Verification items for the finished model (mm, model axes). A direction names the side the tool comes from. Coordinates: 2 decimals unless noted, no trailing zeros. One line per item, written item: value.
```python
from build123d import *

# Parameters (mm, degrees)
F1_DEPTH = 10.16
F2_DEPTH = 12.7


with BuildPart() as f1:
    # F0 (on Front) → F1 (new body)
    with BuildSketch(Plane.XZ):
        with BuildLine():
            ThreePointArc((4.0007179822, 15.285099137), (12.5070249084, 9.654756752), (15.8, 0))
            ThreePointArc((15.8, 0), (-9.7296675451, -12.4488380768), (-3.8169075269, 15.332032381))
            Line((-3.8169075269, 15.332032381), (-3.8169075269, 20.4823272433))
            ThreePointArc((-3.8169075269, 20.4823272433), (-13.314831815, -16.0252852116), (20.834934902, 0))
            ThreePointArc((20.834934902, 0), (16.0849185744, 13.2427303388), (4.0007179822, 20.4472190774))
            Line((4.0007179822, 20.4472190774), (4.0007179822, 15.285099137))
        make_face()
        with BuildLine():
            ThreePointArc((-3.8169075269, 15.332032381), (0.0948538519, 15.7997152742), (4.0007179822, 15.285099137))
            Line((4.0007179822, 15.285099137), (4.0007179822, 20.4472190774))
            ThreePointArc((4.0007179822, 20.4472190774), (2.2310298491, 20.7151398302), (0.4448769206, 20.8301847543))
            Line((0.4448769206, 20.8301847543), (0.1276157176, 20.4966947721))
            Line((0.1276157176, 20.4966947721), (1.8328047784, 18.239185214))
            Line((1.8328047784, 18.239185214), (1.1116877884, 18.239185214))
            Line((1.1116877884, 18.239185214), (-0.2777255205, 20.0982431868))
            Line((-0.2777255205, 20.0982431868), (-0.7255529506, 19.7101260807))
            Line((-0.7255529506, 19.7101260807), (-0.7255529506, 18.239185214))
            Line((-0.7255529506, 18.239185214), (-1.3146182626, 18.239185214))
            Line((-1.3146182626, 18.239185214), (-1.3146182626, 20.7934194205))
            ThreePointArc((-1.3146182626, 20.7934194205), (-2.5704734618, 20.6757630707), (-3.8169075269, 20.4823272433))
            Line((-3.8169075269, 20.4823272433), (-3.8169075269, 15.332032381))
        make_face()
        with BuildLine():
            ThreePointArc((0.4448769206, 20.8301847543), (2.2310298491, 20.7151398302), (4.0007179822, 20.4472190774))
            Line((4.0007179822, 20.4472190774), (4.0007179822, 26.7865807325))
            Line((4.0007179822, 26.7865807325), (-3.8169075269, 26.7865807325))
            Line((-3.8169075269, 26.7865807325), (-3.8169075269, 20.4823272433))
            ThreePointArc((-3.8169075269, 20.4823272433), (-2.5704734618, 20.6757630707), (-1.3146182626, 20.7934194205))
            Line((-1.3146182626, 20.7934194205), (-1.3146182626, 23.8232487851))
            Line((-1.3146182626, 23.8232487851), (-0.7255529506, 23.8232487851))
            Line((-0.7255529506, 23.8232487851), (-0.7255529506, 20.861846369))
            add(Edge.make_bspline(
                [(-0.7255529506, 20.861846369), (-0.7255529506, 20.843060722), (-0.7258157075, 20.8222886334)],
                knots=[0, 0, 0, 0.0956718037, 0.0956718037, 0.0956718037], degree=2))
            ThreePointArc((-0.7258157075, 20.8222886334), (-0.4874986739, 20.8292308407), (-0.2491178041, 20.833445531))
            Line((-0.2491178041, 20.833445531), (1.0140843741, 22.172028671))
            Line((1.0140843741, 22.172028671), (1.7214220586, 22.172028671))
            Line((1.7214220586, 22.172028671), (0.4448769206, 20.8301847543))
        make_face()
    extrude(amount=F1_DEPTH)

    # F0 (on Front) → F2 (join)
    with BuildSketch(Plane.XZ):
        with BuildLine():
            ThreePointArc((4.0007179822, 15.285099137), (12.5070249084, 9.654756752), (15.8, 0))
            ThreePointArc((15.8, 0), (-9.7296675451, -12.4488380768), (-3.8169075269, 15.332032381))
            Line((-3.8169075269, 15.332032381), (-3.8169075269, 20.4823272433))
            ThreePointArc((-3.8169075269, 20.4823272433), (-13.314831815, -16.0252852116), (20.834934902, 0))
            ThreePointArc((20.834934902, 0), (16.0849185744, 13.2427303388), (4.0007179822, 20.4472190774))
            Line((4.0007179822, 20.4472190774), (4.0007179822, 15.285099137))
        make_face()
        with BuildLine():
            ThreePointArc((-3.8169075269, 15.332032381), (0.0948538519, 15.7997152742), (4.0007179822, 15.285099137))
            Line((4.0007179822, 15.285099137), (4.0007179822, 20.4472190774))
            ThreePointArc((4.0007179822, 20.4472190774), (2.2310298491, 20.7151398302), (0.4448769206, 20.8301847543))
            Line((0.4448769206, 20.8301847543), (0.1276157176, 20.4966947721))
            Line((0.1276157176, 20.4966947721), (1.8328047784, 18.239185214))
            Line((1.8328047784, 18.239185214), (1.1116877884, 18.239185214))
            Line((1.1116877884, 18.239185214), (-0.2777255205, 20.0982431868))
            Line((-0.2777255205, 20.0982431868), (-0.7255529506, 19.7101260807))
            Line((-0.7255529506, 19.7101260807), (-0.7255529506, 18.239185214))
            Line((-0.7255529506, 18.239185214), (-1.3146182626, 18.239185214))
            Line((-1.3146182626, 18.239185214), (-1.3146182626, 20.7934194205))
            ThreePointArc((-1.3146182626, 20.7934194205), (-2.5704734618, 20.6757630707), (-3.8169075269, 20.4823272433))
            Line((-3.8169075269, 20.4823272433), (-3.8169075269, 15.332032381))
        make_face()
        with BuildLine():
            ThreePointArc((0.4448769206, 20.8301847543), (2.2310298491, 20.7151398302), (4.0007179822, 20.4472190774))
            Line((4.0007179822, 20.4472190774), (4.0007179822, 26.7865807325))
            Line((4.0007179822, 26.7865807325), (-3.8169075269, 26.7865807325))
            Line((-3.8169075269, 26.7865807325), (-3.8169075269, 20.4823272433))
            ThreePointArc((-3.8169075269, 20.4823272433), (-2.5704734618, 20.6757630707), (-1.3146182626, 20.7934194205))
            Line((-1.3146182626, 20.7934194205), (-1.3146182626, 23.8232487851))
            Line((-1.3146182626, 23.8232487851), (-0.7255529506, 23.8232487851))
            Line((-0.7255529506, 23.8232487851), (-0.7255529506, 20.861846369))
            add(Edge.make_bspline(
                [(-0.7255529506, 20.861846369), (-0.7255529506, 20.843060722), (-0.7258157075, 20.8222886334)],
                knots=[0, 0, 0, 0.0956718037, 0.0956718037, 0.0956718037], degree=2))
            ThreePointArc((-0.7258157075, 20.8222886334), (-0.4874986739, 20.8292308407), (-0.2491178041, 20.833445531))
            Line((-0.2491178041, 20.833445531), (1.0140843741, 22.172028671))
            Line((1.0140843741, 22.172028671), (1.7214220586, 22.172028671))
            Line((1.7214220586, 22.172028671), (0.4448769206, 20.8301847543))
        make_face()
    extrude(amount=F2_DEPTH)


solid = f1.part
```
Item 1: Go/stop test with a flat-tipped pin: P1, Ø1.7, axis at y = -3, z = 22.5, coming from the +X side. Record where the tip stops, or that it passes through.
The answers:
P1: stops at x = 4
Item 2: Draft check along X on faces 1 (the face through (-1.315, -6, 21)), 2 (the face through (4.5, -12.7, 15.4)), 3 (the face through (-3.817, -6, 24)), 4 (the face through (0.37, -6.26, 21.49)). Enter one of: released by +X, released by -X, zero draft, split by the parting line, or undercut.
The answers:
face 1: undercut
face 2: zero draft
face 3: released by -X
face 4: undercut
Item 3: Access from +Z, -Z, +X, -X, +Y, -Y to the whole of each face (thin tool, end or side, straight path). Record for faces 5 (the face through (0.427, -6.261, 19.156)), 6 (the face through (4.001, -6, 24)), 7 (the face through (4.5, 0, 15.4)).
The answers:
face 5: +Y, -Y
face 6: +Z, +X, +Y, -Y
face 7: +Z, -Z, +X, -X, +Y
Item 4: Scan lines: line 1 (Z direction, x = 0, y = -8.5); line 2 (Z direction, x = 10, y = -2.5); line 3 (X direction, y = -5.75, z = -2.5). Record each from-to range of solid material in increasing order.
The answers:
line 1: z = -20.83 to -15.8, 15.8 to 19.73, 21.1 to 26.79
line 2: z = -18.28 to -12.23, 12.23 to 18.28
line 3: x = -20.68 to -15.6, 15.6 to 20.68
